from build123d import *

# Parameters (mm, degrees)
ESBO_O1_W                   = 140
ESBO_O1_H                   = 95
RESSALTO_EXTRUS_O1_DEPTH    = 1.5
ESBO_O2_R                   = 1.5
ESBO_O2_W                   = 40
ESBO_O2_H                   = 3
CORTE_EXTRUS_O1_DEPTH       = 85.647799735
CUT_EXTRUDE12_DEPTH         = 85.607919251
CUT_EXTRUDE12_DEPTH_BACK    = 85.607919251
ESBO_O3_W                   = 3
ESBO_O3_H                   = 31
ESBO_O3_W_2                 = 30
ESBO_O3_H_2                 = 3
RESSALTO_EXTRUS_O2_DEPTH    = 3
CORTE_EXTRUS_O11_DEPTH      = 89.815820663
CORTE_EXTRUS_O11_DEPTH_BACK = 89.815820663
CORTE_EXTRUS_O2_DEPTH       = 89.815820663
CORTE_EXTRUS_O12_DEPTH      = 89.815820663
CORTE_EXTRUS_O12_DEPTH_BACK = 89.815820663
ESBO_O31_R                  = 1.5
CUT_EXTRUDE11_DEPTH         = 89.815820663
CUT_EXTRUDE11_DEPTH_BACK    = 89.815820663
CUT_EXTRUDE14_DEPTH         = 89.777812543
CUT_EXTRUDE14_DEPTH_BACK    = 89.777812543
CUT_EXTRUDE15_DEPTH         = 89.815820663
CUT_EXTRUDE16_DEPTH         = 89.777812543
CUT_EXTRUDE16_DEPTH_BACK    = 89.777812543
SKETCH13_R                  = 1.5
FILLET1_R                   = 5
CUT_EXTRUDE17_DEPTH         = 89.777812543
CUT_EXTRUDE17_DEPTH_BACK    = 89.777812543
SKETCH14_R                  = 1.5


with BuildPart() as part:
    # Esboço1 → Ressalto-extrusão1 (new, symmetric)
    with BuildSketch(Plane.XY):
        Rectangle(ESBO_O1_W, ESBO_O1_H)
    extrude(amount=RESSALTO_EXTRUS_O1_DEPTH, both=True)

    # Esboço2 → Corte-extrusão1 (cut, through all)
    with BuildSketch(Plane.XY.offset(1.5)):
        with Locations((-31.5, -1)):
            Circle(ESBO_O2_R)
        with Locations(Location((31.5, -1, 0), (0, 0, 180))):
            Circle(ESBO_O2_R)
        with Locations((0, -46)):
            Rectangle(ESBO_O2_W, ESBO_O2_H)
        with Locations((0, -1)):
            Rectangle(ESBO_O2_W, ESBO_O2_H)
    extrude(amount=-CORTE_EXTRUS_O1_DEPTH, mode=Mode.SUBTRACT)

    # Sketch9 → Cut-Extrude12 (cut, two sides: drawn at the far end of the back side and taken through both)
    with BuildSketch(Plane.XY.offset(-CUT_EXTRUDE12_DEPTH_BACK)):
        with BuildLine():
            Line((-1.5, -44.5), (1.5, -44.5))
            Line((1.5, -44.5), (1.5, -40.5))
            Line((1.5, -40.5), (2.85, -40.5))
            Line((2.85, -40.5), (2.85, -38.23))
            Line((2.85, -38.23), (1.5, -38.23))
            Line((1.5, -38.23), (1.5, -33.5))
            ThreePointArc((1.5, -33.5), (1.207106781, -32.792893219), (0.5, -32.5))
            Line((0.5, -32.5), (-0.5, -32.5))
            ThreePointArc((-0.5, -32.5), (-1.207106781, -32.792893219), (-1.5, -33.5))
            Line((-1.5, -33.5), (-1.5, -38.23))
            Line((-1.5, -38.23), (-2.85, -38.23))
            Line((-2.85, -38.23), (-2.85, -40.5))
            Line((-2.85, -40.5), (-1.5, -40.5))
            Line((-1.5, -40.5), (-1.5, -44.5))
        make_face()
    extrude(amount=CUT_EXTRUDE12_DEPTH + CUT_EXTRUDE12_DEPTH_BACK, mode=Mode.SUBTRACT)

    # Esboço3 → Ressalto-extrusão2 (add, through all)
    with BuildSketch(Plane.XY.offset(1.5)):
        with Locations((71.5, 0)):
            Rectangle(ESBO_O3_W, ESBO_O3_H)
        with Locations((-71.5, 0)):
            Rectangle(ESBO_O3_W, ESBO_O3_H)
        with Locations((-35, 49)):
            Rectangle(ESBO_O3_W_2, ESBO_O3_H_2)
        with Locations((35, 49)):
            Rectangle(ESBO_O3_W_2, ESBO_O3_H_2)
    extrude(amount=-RESSALTO_EXTRUS_O2_DEPTH)

    # Esboço30 → Corte-extrusão11 (cut, two sides: drawn at the far end of the back side and taken through both)
    with BuildSketch(Plane(origin=(0, 0, -1.5), x_dir=(-1, 0, 0), z_dir=(0, 0, -1)).offset(-CORTE_EXTRUS_O11_DEPTH_BACK)):
        with BuildLine():
            Line((36.5, -21.5), (47.858571571, -21.5))
            ThreePointArc((47.858571571, -21.5), (65, -28.5), (47.858571571, -35.5))
            Line((47.858571571, -35.5), (36.5, -35.5))
            ThreePointArc((36.5, -35.5), (35.085786438, -34.914213562), (34.5, -33.5))
            Line((34.5, -33.5), (34.5, -23.5))
            ThreePointArc((34.5, -23.5), (35.085786438, -22.085786438), (36.5, -21.5))
        make_face()
    extrude(amount=CORTE_EXTRUS_O11_DEPTH + CORTE_EXTRUS_O11_DEPTH_BACK, mode=Mode.SUBTRACT)

    # Esboço4 → Corte-extrusão2 (cut, through all)
    with BuildSketch(Plane.XY.offset(1.5)):
        with BuildLine():
            Line((40, -26.5), (46, -26.5))
            ThreePointArc((46, -26.5), (48, -28.5), (46, -30.5))
            Line((46, -30.5), (40, -30.5))
            ThreePointArc((40, -30.5), (38, -28.5), (40, -26.5))
        make_face()
    extrude(amount=-CORTE_EXTRUS_O2_DEPTH, mode=Mode.SUBTRACT)

    # Esboço31 → Corte-extrusão12 (cut, two sides: drawn at the far end of the back side and taken through both)
    with BuildSketch(Plane(origin=(0, 0, -1.5), x_dir=(-1, 0, 0), z_dir=(0, 0, -1)).offset(-CORTE_EXTRUS_O12_DEPTH_BACK)):
        with Locations((64, -19.5)):
            Circle(ESBO_O31_R)
        with Locations((64, -37.5)):
            Circle(ESBO_O31_R)
        with Locations((31, -19.5)):
            Circle(ESBO_O31_R)
        with Locations((31, -37.5)):
            Circle(ESBO_O31_R)
    extrude(amount=CORTE_EXTRUS_O12_DEPTH + CORTE_EXTRUS_O12_DEPTH_BACK, mode=Mode.SUBTRACT)

    # Sketch8 → Cut-Extrude11 (cut, two sides: drawn at the far end of the back side and taken through both)
    with BuildSketch(Plane(origin=(0, 0, -1.5), x_dir=(-1, 0, 0), z_dir=(0, 0, -1)).offset(-CUT_EXTRUDE11_DEPTH_BACK)):
        with BuildLine():
            Line((-56, 39.75), (-56, 26.75))
            ThreePointArc((-56, 26.75), (-56.439339828, 25.689339828), (-57.5, 25.25))
            Line((-57.5, 25.25), (-60.5, 25.25))
            ThreePointArc((-60.5, 25.25), (-61.560660172, 24.810660172), (-62, 23.75))
            Line((-62, 23.75), (-62, 23.5))
            ThreePointArc((-62, 23.5), (-63.5, 22), (-65, 23.5))
            Line((-65, 23.5), (-65, 23.75))
            ThreePointArc((-65, 23.75), (-65.24500996, 24.571583836), (-65.9, 25.124772708))
            ThreePointArc((-65.9, 25.124772708), (-66.336660027, 25.49356529), (-66.5, 26.041287847))
            Line((-66.5, 26.041287847), (-66.5, 40.458712153))
            ThreePointArc((-66.5, 40.458712153), (-66.336660027, 41.00643471), (-65.9, 41.375227292))
            ThreePointArc((-65.9, 41.375227292), (-65.24500996, 41.928416164), (-65, 42.75))
            Line((-65, 42.75), (-65, 43))
            ThreePointArc((-65, 43), (-63.5, 44.5), (-62, 43))
            Line((-62, 43), (-62, 42.75))
            ThreePointArc((-62, 42.75), (-61.560660172, 41.689339828), (-60.5, 41.25))
            Line((-60.5, 41.25), (-57.5, 41.25))
            ThreePointArc((-57.5, 41.25), (-56.439339828, 40.810660172), (-56, 39.75))
        make_face()
        with BuildLine():
            Line((56, 39.75), (56, 26.75))
            ThreePointArc((56, 26.75), (56.439339828, 25.689339828), (57.5, 25.25))
            Line((57.5, 25.25), (60.5, 25.25))
            ThreePointArc((60.5, 25.25), (61.560660172, 24.810660172), (62, 23.75))
            Line((62, 23.75), (62, 23.5))
            ThreePointArc((62, 23.5), (63.5, 22), (65, 23.5))
            Line((65, 23.5), (65, 23.75))
            ThreePointArc((65, 23.75), (65.24500996, 24.571583836), (65.9, 25.124772708))
            ThreePointArc((65.9, 25.124772708), (66.336660027, 25.49356529), (66.5, 26.041287847))
            Line((66.5, 26.041287847), (66.5, 40.458712153))
            ThreePointArc((66.5, 40.458712153), (66.336660027, 41.00643471), (65.9, 41.375227292))
            ThreePointArc((65.9, 41.375227292), (65.24500996, 41.928416164), (65, 42.75))
            Line((65, 42.75), (65, 43))
            ThreePointArc((65, 43), (63.5, 44.5), (62, 43))
            Line((62, 43), (62, 42.75))
            ThreePointArc((62, 42.75), (61.560660172, 41.689339828), (60.5, 41.25))
            Line((60.5, 41.25), (57.5, 41.25))
            ThreePointArc((57.5, 41.25), (56.439339828, 40.810660172), (56, 39.75))
        make_face()
    extrude(amount=CUT_EXTRUDE11_DEPTH + CUT_EXTRUDE11_DEPTH_BACK, mode=Mode.SUBTRACT)

    # Sketch11 → Cut-Extrude14 (cut, two sides: drawn at the far end of the back side and taken through both)
    with BuildSketch(Plane.XY.offset(-CUT_EXTRUDE14_DEPTH_BACK)):
        with BuildLine():
            Line((33.5, 50.5), (36.5, 50.5))
            Line((36.5, 50.5), (36.5, 46.5))
            Line((36.5, 46.5), (37.85, 46.5))
            Line((37.85, 46.5), (37.85, 44.23))
            Line((37.85, 44.23), (36.5, 44.23))
            Line((36.5, 44.23), (36.5, 39.5))
            ThreePointArc((36.5, 39.5), (36.207106781, 38.792893219), (35.5, 38.5))
            Line((35.5, 38.5), (34.5, 38.5))
            ThreePointArc((34.5, 38.5), (33.792893219, 38.792893219), (33.5, 39.5))
            Line((33.5, 39.5), (33.5, 44.23))
            Line((33.5, 44.23), (32.15, 44.23))
            Line((32.15, 44.23), (32.15, 46.5))
            Line((32.15, 46.5), (33.5, 46.5))
            Line((33.5, 46.5), (33.5, 50.5))
        make_face()
    extrude(amount=CUT_EXTRUDE14_DEPTH + CUT_EXTRUDE14_DEPTH_BACK, mode=Mode.SUBTRACT)

    # Sketch12 → Cut-Extrude15 (cut, through all)
    with BuildSketch(Plane.XY.offset(1.5)):
        with BuildLine():
            Line((-1.5, 20), (-1.5, 35))
            ThreePointArc((-1.5, 35), (0, 36.5), (1.5, 35))
            Line((1.5, 35), (1.5, 20))
            ThreePointArc((1.5, 20), (0, 18.5), (-1.5, 20))
        make_face()
    extrude(amount=-CUT_EXTRUDE15_DEPTH, mode=Mode.SUBTRACT)

    # Sketch13 → Cut-Extrude16 (cut, two sides: drawn at the far end of the back side and taken through both)
    with BuildSketch(Plane.XY.offset(-CUT_EXTRUDE16_DEPTH_BACK)):
        with Locations((12.5, 15.35)):
            Circle(SKETCH13_R)
        with Locations((-12.5, -8.95)):
            Circle(SKETCH13_R)
        with Locations((12.5, -8.95)):
            Circle(SKETCH13_R)
        with Locations((-12.5, 15.35)):
            Circle(SKETCH13_R)
        with BuildLine():
            Line((-10.5, 13.35), (-14.5, 13.35))
            ThreePointArc((-14.5, 13.35), (-15.207106781, 13.057106781), (-15.5, 12.35))
            Line((-15.5, 12.35), (-15.5, 4.15))
            ThreePointArc((-15.5, 4.15), (-15.207106781, 3.442893219), (-14.5, 3.15))
            Line((-14.5, 3.15), (-10.5, 3.15))
            ThreePointArc((-10.5, 3.15), (-9.792893219, 3.442893219), (-9.5, 4.15))
            Line((-9.5, 4.15), (-9.5, 12.35))
            ThreePointArc((-9.5, 12.35), (-9.792893219, 13.057106781), (-10.5, 13.35))
        make_face()
    extrude(amount=CUT_EXTRUDE16_DEPTH + CUT_EXTRUDE16_DEPTH_BACK, mode=Mode.SUBTRACT)

    # Fillet1
    fillet1_edges = [part.edges().sort_by_distance(p)[0] for p in [
        (-70, 47.5, 0),
        (70, 47.5, 0),
    ]]
    fillet(fillet1_edges, radius=FILLET1_R)

    # Sketch14 → Cut-Extrude17 (cut, two sides: drawn at the far end of the back side and taken through both)
    with BuildSketch(Plane.XY.offset(-CUT_EXTRUDE17_DEPTH_BACK)):
        with Locations((-29.75, 37.9)):
            Circle(SKETCH14_R)
        with Locations((-40.25, 37.9)):
            Circle(SKETCH14_R)
    extrude(amount=CUT_EXTRUDE17_DEPTH + CUT_EXTRUDE17_DEPTH_BACK, mode=Mode.SUBTRACT)


solid = part.part
Verification items for the finished model (mm, model axes). A direction names the side the tool comes from. Coordinates: 2 decimals unless noted, no trailing zeros. Write each loop counter-clockwise with the first axis right and the second up, starting at its lowest first coordinate (ties: lowest second). Pieces come first, ordered by that corner, then holes. Notation, with made-up numbers: (56.25, 35.5) -> (72.25, 35.5) arc R18 cw to (72.25, 63.5) -> close; hole circle Ø7 at (84, -4). An arc over 180 degrees is marked (long way). One line per item, written item: value. Start each with the question number.
Q1. Cross-section at C-C on z = -0.35. State how many separate pieces and enclosed holes the cut face has, and give its area (3 significant figures).
Q2. Mould release check, pull along X, two halves, no side actions. Record for faces 5 (the flat face through (-1.5, -36, 0)), 6 (the flat face through (43, 50.5, 0)), 7 (the flat face through (-70, 29, 0)): pulls with the +X half, pulls with the -X half, needs draft (parallel to the pull), parting line crosses it, or undercut.
Q3. Go/stop test with flat-tipped pins: P1, Ø1.1, axis at y = -39, z = 0, coming from the -X side; P2, Ø0.9, axis at y = -35, z = 0, coming from the +X side. Record where each tip stops, or that it passes through.
Q4. Thickness scan on L1, parallel to Y at x = -12.5, z = -0.35; L2, parallel to Y at x = 12.5, z = 0.3; L3, parallel to X at y = -28.5, z = 0.45. Record the ranges inside material, lowest first. Write a range as from..to.
Q5. Cross-section at B-B on x = 63.5. Enter the section's corners in (y, z), and give its area (4 significant figures).
Q6. Cross-section at D-D on x = -44.5. Enter the section's corners in (y, z).
Q7. Cross-section at A-A on x = -12.5. Enter the section's corners in (y, z), and give its area (3 significant figures).
Q8. Access from +Z, -Z, +X, -X, +Y, -Y to the whole of each face (thin tool, end or side, straight path). Record for faces 1 (the flat face through (-50, 49, 0)), 2 (the cylindrical face through (0, 18.5, 0)), 3 (the flat face through (57, 47.5, 0)), 4 (the flat face through (20, 49, 0)).
Checked values:
1. separate pieces: 1
1. enclosed holes: 19
1. area: 12,300 mm²
2. face 5: undercut
2. face 6: needs draft
2. face 7: pulls with the -X half
3. P1: stops at x = -70
3. P2: stops at x = 70
4. L1: y = -44.5..-10.45, -7.45..-2.5, 0.5..3.15, 13.35..13.85, 16.85..47.5
4. L2: y = -44.5..-10.45, -7.45..-2.5, 0.5..13.85, 16.85..47.5
4. L3: x = -70..-65, -34.5..38, 48..70
5. outline: (-47.5, -1.5) -> (22, -1.5) -> (22, 1.5) -> (-47.5, 1.5) -> close; (44.5, -1.5) -> (47.5, -1.5) -> (47.5, 1.5) -> (44.5, 1.5) -> close
5. area: 217.5 mm²
6. outline: (-47.5, -1.5) -> (-35.5, -1.5) -> (-35.5, 1.5) -> (-47.5, 1.5) -> close; (-21.5, -1.5) -> (50.5, -1.5) -> (50.5, 1.5) -> (-21.5, 1.5) -> close
7. outline: (-44.5, -1.5) -> (-10.45, -1.5) -> (-10.45, 1.5) -> (-44.5, 1.5) -> close; (-7.45, -1.5) -> (-2.5, -1.5) -> (-2.5, 1.5) -> (-7.45, 1.5) -> close; (0.5, -1.5) -> (3.15, -1.5) -> (3.15, 1.5) -> (0.5, 1.5) -> close; (13.35, -1.5) -> (13.85, -1.5) -> (13.85, 1.5) -> (13.35, 1.5) -> close; (16.85, -1.5) -> (47.5, -1.5) -> (47.5, 1.5) -> (16.85, 1.5) -> close
7. area: 218 mm²
8. face 1: +Z, -Z, -X, +Y
8. face 2: +Z, -Z
8. face 3: +Z, -Z, +X, +Y
8. face 4: +Z, -Z, +Y
